```python
from build123d import *

# Parameters (mm, degrees)
BASE_FLANGE1_DEPTH               = 793.75
E_0_25_DIAMETER_HOLE1_D          = 6.35
F_10_0_1935_DIAMETER_HOLE1_D     = 4.9149
FILLET1_R                        = 3.175
F_17_64_0_26563_DIAMETER_HOLE2_D = 6.747002
F_10_0_1935_DIAMETER_HOLE2_D     = 4.9149


# Sheet-metal steps are written as plain solids
with BuildPart() as part:
    # Sketch1 → Base-Flange1 (new, symmetric)
    with BuildSketch(Plane.XY):
        with BuildLine():
            Line((0, 0), (-34.925, 0))
            ThreePointArc((-34.925, 0), (-39.415128061, 1.859871939), (-41.275, 6.35))
            Line((-41.275, 6.35), (-41.275, 41.275))
            Line((-41.275, 41.275), (-38.1, 41.275))
            Line((-38.1, 41.275), (-38.1, 6.35))
            ThreePointArc((-38.1, 6.35), (-37.17006403, 4.10493597), (-34.925, 3.175))
            Line((-34.925, 3.175), (0, 3.175))
            Line((0, 3.175), (0, 0))
        make_face()
    extrude(amount=BASE_FLANGE1_DEPTH, both=True)

    # E (0.25) Diameter Hole1 (through all)
    with Locations(Plane(origin=(0, 3.175, 0), x_dir=(1, 0, 0), z_dir=(0, 1, 0))):
        with Locations((-12.7, 6.35), (-12.7, -6.35), (-12.7, 234.95), (-12.7, 222.25), (-12.7, 463.55), (-12.7, 450.85), (-12.7, 692.15), (-12.7, 679.45), (-12.7, -222.25), (-12.7, -234.95), (-12.7, -450.85), (-12.7, -463.55), (-12.7, -679.45), (-12.7, -692.15)):
            Hole(E_0_25_DIAMETER_HOLE1_D / 2)

    # #10 (0.1935) Diameter Hole1 (through all)
    with Locations(Plane(origin=(0, 3.175, 0), x_dir=(1, 0, 0), z_dir=(0, 1, 0))):
        with Locations((-12.7, -765.175), (-12.7, -781.685), (-12.7, 781.685), (-12.7, 765.175)):
            Hole(F_10_0_1935_DIAMETER_HOLE1_D / 2)

    # Fillet1
    fillet1_edges = [part.edges().sort_by_distance(p)[0] for p in [
        (0, 1.5875, 793.75),
        (0, 1.5875, -793.75),
        (-39.6875, 41.275, 793.75),
        (-39.6875, 41.275, -793.75),
    ]]
    fillet(fillet1_edges, radius=FILLET1_R)

    # 17/64 (0.26563) Diameter Hole2 (through all)
    with Locations(Plane(origin=(0, 3.175, 0), x_dir=(1, 0, 0), z_dir=(0, 1, 0))):
        with Locations((-9.525, 365.4425), (-9.525, -365.4425)):
            Hole(F_17_64_0_26563_DIAMETER_HOLE2_D / 2)

    # #10 (0.1935) Diameter Hole2 (through all)
    with Locations(Plane(origin=(-38.1, 0, 0), x_dir=(0, 0, -1), z_dir=(1, 0, 0))):
        with Locations((-771.525, 28.575), (771.525, 28.575)):
            Hole(F_10_0_1935_DIAMETER_HOLE2_D / 2)


solid = part.part
```
Read the model definition and answer for the solid it produces. Units are mm, in the model's axes. A direction names the side the tool comes from. Round coordinates to 2 decimals unless told otherwise and drop trailing zeros. Loops run counter-clockwise (first coordinate to the right, second up) from the corner with the lowest first, then second, coordinate; pieces in that order, holes last. Notation, with made-up numbers: (55, 63.5) -> (72, 63.5) arc R21 cw to (72, 76.5) -> close; hole circle Ø5 at (-37.75, 48). An arc over 180 degrees is marked (long way). One line per item, written item: value.
1) Flat-ended cylindrical pins translate along their axes: P1, Ø4, axis at x = -33.5, z = -401.5, coming from the +Y side; P2, Ø4.5, axis at x = -12.7, z = 765.175, coming from the -Y side. Find the tip coordinate at first contact, or state that the pin passes through.
Answer list:
P1: stops at y = 3.23
P2: passes through
2) Consider L1, parallel to X at y = 0.9, z = 692.15 (3 decimals); L2, parallel to Y at x = -18, z = 635.5 (3 decimals); L3, parallel to X at y = 32, z = 345.5 (3 decimals). Determine where each line is inside the solid, lowest interval first. Write a range as [from, to].
Answer list:
L1: x = [-38.184, -15.875], [-9.525, 0]
L2: y = [0, 3.175]
L3: x = [-41.275, -38.1]
3) For faces 1 (the face through (-18, 3.175, 11)), 2 (the face through (-41.275, 24, 11)), determine the directions among +Z, -Z, +X, -X, +Y, -Y from which every point of the face is accessible in a straight line to the end or side of a thin tool.
Answer list:
face 1: +Z, -Z, +X, +Y
face 2: +Z, -Z, -X, +Y, -Y
4) A cutting plane is placed at A-A (z = -33). Determine the outline of the cut face in (x, y) (3 decimals).
Answer list:
outline: (-41.275, 6.35) arc R6.35 ccw to (-34.925, 0) -> (0, 0) -> (0, 3.175) -> (-34.925, 3.175) arc R3.175 cw to (-38.1, 6.35) -> (-38.1, 41.275) -> (-41.275, 41.275) -> close
